Can you work these out from the model? Positions are in its coordinate system, mm. A direction names the side the tool comes from. Coordinates: 2 decimals unless noted, no trailing zeros. Write each loop counter-clockwise with the first axis right and the second up, starting at its lowest first coordinate (ties: lowest second). Pieces come first, ordered by that corner, then holes. Notation, with made-up numbers: (9, 30) -> (49, 30) arc R17 cw to (49, 62) -> close; hole circle Ø1 at (39, 63.5). An arc over 180 degrees is marked (long way). Answer as CSV lines item,"result". Start each with the question number.
```python
from build123d import *

# Parameters (mm, degrees)
SKETCH1_W           = 15
SKETCH1_H           = 15
BOSS_EXTRUDE1_DEPTH = 5
SKETCH2_W           = 9.136161194
SKETCH2_H           = 15
CUT_EXTRUDE1_DEPTH  = 2
CUT_EXTRUDE2_DEPTH  = 12


with BuildPart() as part:
    # Sketch1 → Boss-Extrude1 (new body)
    with BuildSketch(Plane.XY):
        Rectangle(SKETCH1_W, SKETCH1_H)
    extrude(amount=BOSS_EXTRUDE1_DEPTH)

    # Sketch2 → Cut-Extrude1 (cut)
    with BuildSketch(Plane.XY.offset(5)):
        Rectangle(SKETCH2_W, SKETCH2_H)
    extrude(amount=-CUT_EXTRUDE1_DEPTH, mode=Mode.SUBTRACT)

    # Sketch3 → Cut-Extrude2 (cut)
    with BuildSketch(Plane.XY.offset(3)):
        with BuildLine():
            Line((-1.7, 3.8), (-1.7, -3.8))
            ThreePointArc((-1.7, -3.8), (0, -5.5), (1.7, -3.8))
            Line((1.7, -3.8), (1.7, 3.8))
            ThreePointArc((1.7, 3.8), (0, 5.5), (-1.7, 3.8))
        make_face()
    extrude(amount=-CUT_EXTRUDE2_DEPTH, mode=Mode.SUBTRACT)


solid = part.part
```
Q1. Imagine slicing it at B-B (x = -1.5). Write out the boundary of the cut face in (y, z), then the cut area to 3 significant figures.
Q2. If we mould it in two halves opening along X, with no side actions, what happens to faces 4 (the face through (-4.568, 0, 4)), 5 (the face through (-7.5, 0, 2)), 6 (the face through (0, 7.5, 2))? For each: released by +X, released by -X, zero draft, split by the parting line, or undercut.
Q3. Imagine slicing it at D-D (z = 1.65). Write out the boundary of the cut face in (x, y), then the cut area to 3 significant figures.
Q4. Which directions (+Z, -Z, +X, -X, +Y, -Y) give clear straight access to the entire face, cutting with the end or side of a thin tool? Please do faces 1 (the face through (1.7, 0, 2)), 2 (the face through (7.5, 0, 2)), 3 (the face through (2, 0, 3)).
Q5. I need wall thicknesses on L1, parallel to X at y = 2, z = 0.25; L2, parallel to X at y = 4, z = 3.85; L3, parallel to Z at x = 3.75, y = 2.25. Which ranges of each line are inside material? Lowest first, please.
Q6. For pin 1 (4.5 mm diameter, centred on x = -2, y = 2.5, fed in from +Z), with a flat end and sliding along its axis, tell me the tip position at first contact or that it passes through.
Q7. Imagine slicing it at A-A (y = -1). Write out the boundary of the cut face in (x, z), then the cut area to 3 significant figures.
Q8. Imagine slicing it at C-C (z = 4.6). Write out the boundary of the cut face in (x, y), then the cut area to 3 significant figures.
Entries:
1,outline,"(-7.5, 0) -> (-4.6, 0) -> (-4.6, 3) -> (-7.5, 3) -> close; (4.6, 0) -> (7.5, 0) -> (7.5, 3) -> (4.6, 3) -> close"
1,area,"17.4 mm2"
2,face 4,"undercut"
2,face 5,"released by -X"
2,face 6,"zero draft"
3,outline,"(-7.5, -7.5) -> (7.5, -7.5) -> (7.5, 7.5) -> (-7.5, 7.5) -> close; hole (-1.7, -3.8) arc R1.7 ccw to (1.7, -3.8) -> (1.7, 3.8) arc R1.7 ccw to (-1.7, 3.8) -> close"
3,area,"190 mm2"
4,face 1,"+Z, -Z"
4,face 2,"+Z, -Z, +X, +Y, -Y"
4,face 3,"+Z, +Y, -Y"
5,L1,"-7.5 to -1.7, 1.7 to 7.5"
5,L2,"-7.5 to -4.57, 4.57 to 7.5"
5,L3,"0 to 3"
6,pin 1,"z = 3"
7,outline,"(-7.5, 0) -> (-1.7, 0) -> (-1.7, 3) -> (-4.57, 3) -> (-4.57, 5) -> (-7.5, 5) -> close; (1.7, 0) -> (7.5, 0) -> (7.5, 5) -> (4.57, 5) -> (4.57, 3) -> (1.7, 3) -> close"
7,area,"46.5 mm2"
8,outline,"(-7.5, -7.5) -> (-4.57, -7.5) -> (-4.57, 7.5) -> (-7.5, 7.5) -> close; (4.57, -7.5) -> (7.5, -7.5) -> (7.5, 7.5) -> (4.57, 7.5) -> close"
8,area,"88.0 mm2"
